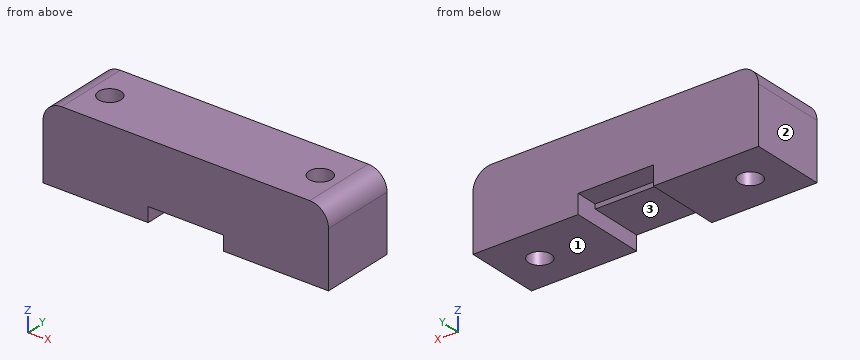
Autodesk Inventor part; units mm, degrees
ref_plane "YZ Plane" through (0, 0, 0) normal (1, 0, 0) x (0, 1, 0)
ref_plane "XZ Plane" through (0, 0, 0) normal (0, 1, 0) x (-1, 0, 0)
ref_plane "XY Plane" through (0, 0, 0) normal (0, 0, 1) x (1, 0, 0)
sketch "Sketch1" plane through (0, 0, 0) normal (0, 0, 1) x (1, 0, 0)
  line L0 (-38, 10) -> (38, 10)
  line L1 (38, 10) -> (38, -10)
  line L2 (38, -10) -> (-38, -10)
  line L3 (-38, -10) -> (-38, 10)
  point P0 (0, 0)
  point P1 (-38, 0)
  point P2 (0, 10)
  dimension "d0" = 76
  dimension "d1" = 20
extrude "Extrusion1" add sketch "Sketch1" along normal blind 20
sketch "Sketch6" plane through (0, 0, 0) normal (1, 0, 0) x (0, 1, 0)
  line L0 (12, 5.4) -> (4.47, 5.4)
  line L1 (4.47, 4.175) -> (-0.23, 4.175)
  line L2 (10, 0) -> (10, 20)
  line L3 (-10, 0) -> (-10, 20)
  line L4 (10, 5.1) -> (4.17, 5.1)
  line L5 (4.17, 5.1) -> (4.17, 3.875)
  line L6 (4.17, 3.875) -> (-10, 3.875)
  line L7 (10, 0) -> (-10, 0)
  point P0 (0, 0)
  point P1 (4.17, 0)
  dimension "d16" = 0.3
  dimension "d17" = 0.3
  dimension "d18" = 0.3
extrude "Extrusion5" cut sketch "Sketch6" along normal mid plane 20
sketch "Sketch7" plane through (0, 0, 20) normal (0, 0, 1) x (1, 0, 0)
  line L0 (-38, 10) -> (-38, -10)
  line L1 (38, -10) -> (38, 10)
  point P0 (0, 0)
  point P1 (28, 0)
  point P2 (-28, 0)
  dimension "d21" = 10
  dimension "d22" = 10
hole "Hole1" at (-28, 0, 20) at (28, 0, 20) direction (0, 0, -1) diameter 6 end through all
fillet "Fillet3" radius 5 2 edges at (-38, 0, 20) (38, 0, 20)
properties part number "0008-30-013"
Input: part model. Units: mm. Frame: model coordinates. Face numbers are marked on the shaded views. Coordinates: 2 decimals unless noted, no trailing zeros. Write each loop counter-clockwise with the first axis right and the second up, starting at its lowest first coordinate (ties: lowest second). Pieces come first, ordered by that corner, then holes. Notation, with made-up numbers: (71.5, 26.25) - (105.5, 26.25) arc R22 cw to (105.5, 63.25) - close; hole circle Ø8 at (66, 11.25). An arc over 180 degrees is marked (long way). Put each result on its own line as item: value. Start each with the question number.
1) Cut plane A-A (x = 28). Return the cut outline in (y, z).
2) Cut plane B-B (y = 0). Return the cut outline in (x, z) (3 decimals), plus the area to 3 significant figures.
3) Cut plane D-D (y = -7.5). Return the cut outline in (x, z) (3 decimals), plus the area to 3 significant figures.
4) Cut plane C-C (z = 14.25). Return the cut outline in (x, y), plus the area to 3 significant figures.
5) Mould query, pull axis X, two halves, no side actions, for the marked faces 1, 2 and 3. Classes: pulls with the +X half, pulls with the -X half, needs draft (parallel to the pull), parting line crosses it, or undercut.
6) Contact query for flat-ended pins moving along their axis: pin 1 (7 mm diameter, centred on x = 4.5, y = -3.5, fed in from -Z) (3 decimals); pin 2 (4 mm diameter, centred on x = 11.5, y = -2.5, fed in from -Z); pin 3 (1 mm diameter, centred on x = -0.5, z = 4.5, fed in from +Y). Output: stop coordinate, or through.
7) Ray query, L1, parallel to Y at x = -28, z = 6; L2, parallel to X at y = -0.75, z = 9.5; L3, parallel to X at y = -1, z = 1.75. Return the intervals inside material, ascending.
Resolved:
1. outline: (-10, 0) - (-3, 0) - (-3, 20) - (-10, 20) - close; (3, 0) - (10, 0) - (10, 20) - (3, 20) - close
2. outline: (-38, 0) - (-31, 0) - (-31, 20) - (-33, 20) arc R5 ccw to (-38, 15) - close; (-25, 0) - (-10, 0) - (-10, 3.875) - (10, 3.875) - (10, 0) - (25, 0) - (25, 20) - (-25, 20) - close; (31, 0) - (38, 0) - (38, 15) arc R5 ccw to (33, 20) - (31, 20) - close
2. area: 1,190 mm2
3. outline: (-38, 0) - (-10, 0) - (-10, 3.875) - (10, 3.875) - (10, 0) - (38, 0) - (38, 15) arc R5 ccw to (33, 20) - (-33, 20) arc R5 ccw to (-38, 15) - close
3. area: 1,430 mm2
4. outline: (-38, -10) - (38, -10) - (38, 10) - (-38, 10) - close; hole circle Ø6 at (-28, 0); hole circle Ø6 at (28, 0)
4. area: 1,460 mm2
5. face 1: needs draft
5. face 2: pulls with the -X half
5. face 3: undercut
6. pin 1: stops at z = 3.875
6. pin 2: stops at z = 0
6. pin 3: stops at y = 4.17
7. L1: y = -10 to -3, 3 to 10
7. L2: x = -38 to -30.9, -25.1 to 25.1, 30.9 to 38
7. L3: x = -38 to -30.83, -25.17 to -10, 10 to 25.17, 30.83 to 38
